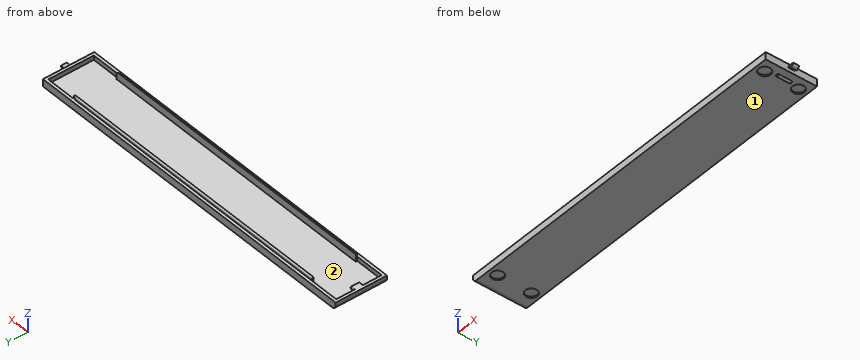
from build123d import *

# Parameters (mm, degrees)
F0_W         = 35
F0_H         = 5
F1_DEPTH     = 120
F2_T         = -2
F4_DEPTH     = 3
F6_DEPTH     = 2
F7_T1_DEPTH  = 10.0971618345
F8_W         = 196
F8_H         = 5
F9_DEPTH     = 1
F10_W        = 196
F10_H        = 2
F10_H_2      = 3
F11_DEPTH    = 1
F12_T1_DEPTH = 9.5
F13_R        = 0.99999
F14_R        = 0.5
F15_R        = 4
F16_DEPTH    = 1
F17_W        = 2
F17_H        = 10
F18_DEPTH    = 1
F19_R        = 0.99999
F20_R        = 3


# Not quite as in the source:
# - a fillet or chamfer that OpenCascade refuses, or shapes differently, is made with other operations: its cross-section is extruded or revolved along the edge and cut away or added
# - a fillet or chamfer is up to 0.001 mm smaller than in the source, because OpenCascade refuses the exact size


with BuildPart() as f1:
    # F0 (on Right) → F1 (new body, symmetric)
    with BuildSketch(Plane.YZ):
        Rectangle(F0_W, F0_H)
    extrude(amount=F1_DEPTH, both=True)

    # F2
    f2_openings = [f1.faces().sort_by_distance(p)[0] for p in [
        (0, 0, 2.5),
    ]]
    offset(amount=F2_T, openings=f2_openings)

    # F3 (on Front) → F4 (join, symmetric)
    with BuildSketch(Plane.XZ):
        Polygon((-114, 2.5), (-118, 2.5), (-118, 0.5), (-116, 0.5), align=None)
    extrude(amount=F4_DEPTH, both=True)

    # F5 (on Front) → F6 (join, symmetric)
    with BuildSketch(Plane.XZ):
        Polygon((123.9, 1), (120, 1), (120, 0), (121.9, 0), (123.9, 0), align=None)
        Polygon((121.9, -1), (123.9, 0), (121.9, 0), align=None)
    extrude(amount=F6_DEPTH, both=True)

    # F7: fillet of radius 2 on 1 edges, made by hand

    # F7_s2 → F7_t1 (cut)
    with BuildSketch(Plane.XZ.offset(-5.0485809173)):
        with BuildLine():
            ThreePointArc((123.9, 1), (123.5488845703, 0.09023972), (122.8093065335, -0.5453467333))
            Line((122.8093065335, -0.5453467333), (123.9, 0))
            Line((123.9, 0), (123.9, 1))
        make_face()
    extrude(amount=F7_T1_DEPTH, mode=Mode.SUBTRACT)

    # F8 (on face) → F9 (join)
    with BuildSketch(Plane(origin=(0, -15.5, 0), x_dir=(-1, 0, 0), z_dir=(0, 1, 0))):
        with Locations((0, 2)):
            Rectangle(F8_W, F8_H)
    extrude(amount=F9_DEPTH)

    # F10 (on face) → F11 (join)
    with BuildSketch(Plane.XZ.offset(-15.5)):
        with Locations((0, 3.5)):
            Rectangle(F10_W, F10_H)
        with Locations((0, 1)):
            Rectangle(F10_W, F10_H_2)
    extrude(amount=F11_DEPTH)

    # F12: fillet of radius 5 on 2 edges, made by hand

    # F12_s2 → F12_t1 (cut)
    with BuildSketch(Plane.XY.offset(2.5)):
        with BuildLine():
            ThreePointArc((95, 15.5), (96.5811388301, 15.2434164903), (98, 14.5))
            Line((98, 14.5), (98, 15.5))
            Line((98, 15.5), (95, 15.5))
        make_face()
        with BuildLine():
            ThreePointArc((95, -15.5), (96.5811388301, -15.2434164903), (98, -14.5))
            Line((98, -14.5), (98, -15.5))
            Line((98, -15.5), (95, -15.5))
        make_face()
    extrude(amount=F12_T1_DEPTH, mode=Mode.SUBTRACT)

    # F13 (radius 1 in the source; OpenCascade refuses exactly that, so slightly less here)
    f13_edges = [f1.edges().sort_by_distance(p)[0] for p in [
        (-1.5, -15.5, 4.5),
        (-1.5, 15.5, 4.5),
    ]]
    fillet(f13_edges, radius=F13_R)

    # F14
    f14_edges = [f1.edges().sort_by_distance(p)[0] for p in [
        (-114, 0, 2.5),
        (-116, -3, 2.5),
        (-116, 3, 2.5),
    ]]
    fillet(f14_edges, radius=F14_R)

    # F15 (on face) → F16 (cut)
    with BuildSketch(Plane(origin=(0, 0, -2.5), x_dir=(1, 0, 0), z_dir=(0, 0, -1))):
        with Locations((-107, 11.5)):
            Circle(F15_R)
        with Locations((-107, -11.5)):
            Circle(F15_R)
        with Locations((112, -11.5)):
            Circle(F15_R)
        with Locations((112, 11.5)):
            Circle(F15_R)
    extrude(amount=-F16_DEPTH, mode=Mode.SUBTRACT)

    # F17 (on face) → F18 (join)
    with BuildSketch(Plane(origin=(0, 0, -2.5), x_dir=(1, 0, 0), z_dir=(0, 0, -1))):
        with Locations((114, 0)):
            Rectangle(F17_W, F17_H)
    extrude(amount=F18_DEPTH)

    # F19 (radius 1 in the source; OpenCascade refuses exactly that, so slightly less here)
    f19_edges = [f1.edges().sort_by_distance(p)[0] for p in [
        (114, -5, -3.5),
        (115, 0, -3.5),
        (114, 5, -3.5),
        (113, 0, -3.5),
    ]]
    fillet(f19_edges, radius=F19_R)

    # F20
    f20_edges = [f1.edges().sort_by_distance(p)[0] for p in [
        (-120, 0, -2.5),
    ]]
    fillet(f20_edges, radius=F20_R)


solid = f1.part
CAD build for the part. Positions are in the model's coordinates, mm. Face numbers are marked on the shaded views. Round coordinates to 2 decimals unless told otherwise and drop trailing zeros. Write each loop counter-clockwise with the first axis right and the second up, starting at its lowest first coordinate (ties: lowest second). Pieces come first, ordered by that corner, then holes. Notation, with made-up numbers: M 0,58.25 L 41,58.25 A24 cw 41,90.25 Z; hole C 75,21.25 d11. An arc over 180 degrees is marked long. Use a Markdown table: item, result. Add a question column.
1. Flat gauge pins, fed straight in: P1, Ø1, axis at y = 0.5, z = -1, coming from the -X side; P2, Ø3, axis at y = -5, z = 0.5, coming from the +X side; P3, Ø1.2, axis at x = 121, y = 0, coming from the +Z side. Where does each tip first touch, or does it go through?
2. Drill centre lines: probe 1 along Y at (x, z) = (112, -2); probe 2 along X at (y, z) = (-15, 0.75); probe 3 along Y at (x, z) = (59.5, 1.5). Where is each one in solid material? Low to high.
3. Slice it at A-A on y = -11.5. Give the cut face in (x, z), then the cut area to 3 significant figures.
4. Slice it at D-D on y = 9.5. Give the cut face in (x, z), then the cut area to 3 significant figures.
5. Slice it at C-C on x = -107. Give the cut face in (y, z), then the cut area to 3 significant figures.
6. Pull direction X, two halves, no side cores. Call the marked faces 1 and 2: released by +X, released by -X, zero draft, split by the parting line, or undercut.
Reply:
| question | item | result |
|---|---|---|
| 1 | P1 | stops at x = -119.83 |
| 1 | P2 | stops at x = 120 |
| 1 | P3 | stops at z = 1 |
| 2 | probe 1 | y = -17.5 to -15.5, -7.5 to 7.5, 15.5 to 17.5 |
| 2 | probe 2 | x = -120 to -118, -98 to 98, 118 to 120 |
| 2 | probe 3 | y = -17.5 to -14.5, 14.5 to 17.5 |
| 3 | outline | M -120,0.5 A3 ccw -117,-2.5 L -111,-2.5 L -111,-1.5 L -103,-1.5 L -103,-2.5 L 108,-2.5 L 108,-1.5 L 116,-1.5 L 116,-2.5 L 120,-2.5 L 120,2.5 L 118,2.5 L 118,-0.5 L -118,-0.5 L -118,2.5 L -120,2.5 Z |
| 3 | area | 474 mm^2 |
| 4 | outline | M -120,0.5 A3 ccw -117,-2.5 L -110.46,-2.5 L -110.46,-1.5 L -103.54,-1.5 L -103.54,-2.5 L 108.54,-2.5 L 108.54,-1.5 L 115.46,-1.5 L 115.46,-2.5 L 120,-2.5 L 120,2.5 L 118,2.5 L 118,-0.5 L -118,-0.5 L -118,2.5 L -120,2.5 Z |
| 4 | area | 476 mm^2 |
| 5 | outline | M -17.5,-2.5 L -15.5,-2.5 L -15.5,-1.5 L -7.5,-1.5 L -7.5,-2.5 L 7.5,-2.5 L 7.5,-1.5 L 15.5,-1.5 L 15.5,-2.5 L 17.5,-2.5 L 17.5,2.5 L 15.5,2.5 L 15.5,-0.5 L -15.5,-0.5 L -15.5,2.5 L -17.5,2.5 Z |
| 5 | area | 66.0 mm^2 |
| 6 | face 1 | zero draft |
| 6 | face 2 | undercut |
